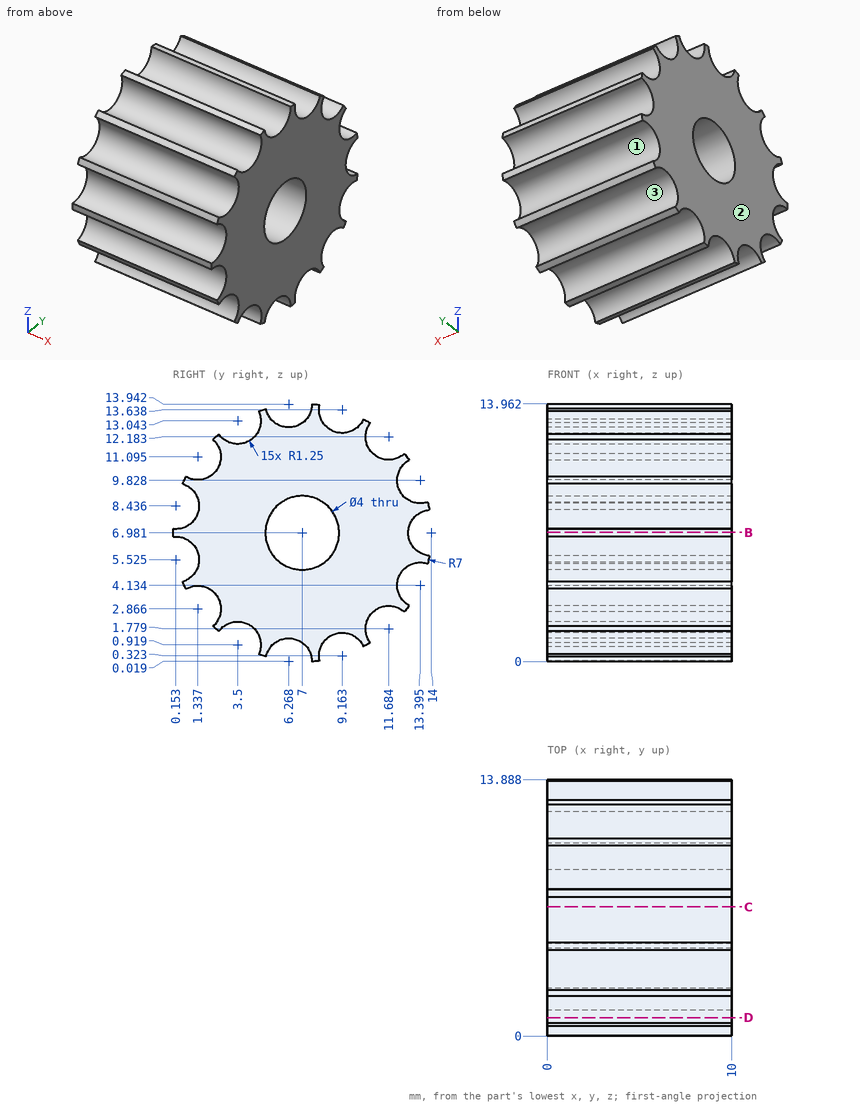
Could you check a few things on this drawing? It's one solid part, dimensions in mm from its lowest x, y, z. Coordinates: 2 decimals unless noted, no trailing zeros. Order: outer loops, then holes, each group sorted by start corner. A loop starts at its lowest first (then second) coordinate and runs counter-clockwise, first axis right, second up. Notation, with made-up numbers: M -29.5,8 L 23.5,8 A23 cw 23.5,28 Z; hole C -17,57.25 d1. An arc over 180 degrees is marked long. Use a Markdown table: item, result. Add a question column.
Q1. I'm going to push flat-ended pins straight in: pin 1 (1.5 mm diameter, centred on x = 2, y = 10, fed in from -Z); pin 2 (3 mm diameter, centred on x = 4, z = 9.5, fed in from +Y); pin 3 (3 mm diameter, centred on y = 7, z = 6.98, fed in from -X). Where does each tip first touch, or does it pass through?
Q2. I want a section at D-D on y = 1. List the corners of the cut face in (x, z) for me (1 decimal).
Q3. I want a section at B-B on z = 7. List the corners of the cut face in (x, y) for me.
Q4. If I drill on L1, parallel to Z at x = 5, y = 12.5 (1 decimal); L2, parallel to Z at x = 4.5, y = 12.25 (1 decimal); L3, parallel to Y at x = 1.25, z = 8.75 (1 decimal), over which ranges is the centre line in solid material (lowest first)?
Q5. We'd pull the mould along Z, two halves only. Please class the marked faces 1, 2 and 3: pulls with the +Z half, pulls with the -Z half, needs draft (parallel to the pull), parting line crosses it, or undercut.
Q6. I want a section at C-C on y = 7. List the corners of the cut face in (x, z) for me.
Checked values:
| question | item | result |
|---|---|---|
| 1 | pin 1 | z = 0.81 |
| 1 | pin 2 | y = 13.89 |
| 1 | pin 3 | through |
| 2 | outline | M 0,4.1 L 10,4.1 L 10,4.6 L 0,4.6 Z; M 0,6.4 L 10,6.4 L 10,7.5 L 0,7.5 Z; M 0,9.4 L 10,9.4 L 10,9.9 L 0,9.9 Z |
| 3 | outline | M 0,0 L 10,0 L 10,5 L 0,5 Z; M 0,9 L 10,9 L 10,12.75 L 0,12.75 Z |
| 4 | L1 | 2.7 to 3.3, 5 to 9, 10.7 to 11.2 |
| 4 | L2 | 2.9 to 3.6, 4.6 to 9.3, 10.3 to 11.1 |
| 4 | L3 | 1.4 to 6.1, 7.9 to 12.8 |
| 5 | face 1 | undercut |
| 5 | face 2 | needs draft |
| 5 | face 3 | undercut |
| 6 | outline | M 0,1.03 L 10,1.03 L 10,4.98 L 0,4.98 Z; M 0,8.98 L 10,8.98 L 10,12.93 L 0,12.93 Z |
